Autodesk Inventor part; units mm, degrees
ref_plane "YZ Plane" through (0, 0, 0) normal (1, 0, 0) x (0, 1, 0)
ref_plane "XZ Plane" through (0, 0, 0) normal (0, 1, 0) x (-1, 0, 0)
ref_plane "XY Plane" through (0, 0, 0) normal (0, 0, 1) x (1, 0, 0)
sketch "Sketch1" plane through (0, 0, 0) normal (0, 0, 1) x (1, 0, 0)
  line L0 (8, 0.0718) -> (2, 3.5359)
  line L1 (2, 3.5359) -> (2, 10.4641)
  line L2 (2, 10.4641) -> (8, 13.9282)
  line L3 (8, 13.9282) -> (14, 10.4641)
  line L4 (14, 10.4641) -> (14, 3.5359)
  line L5 (14, 3.5359) -> (8, 0.0718)
  point P0 (0, 0)
  point P1 (8, 7)
  dimension "d1" = 12
extrude "Extrusion1" add sketch "Sketch1" along normal blind 18
sketch "Sketch2" plane through (0, 0, 0) normal (0, 0, -1) x (-1, 0, 0)
  circle A0 centre (-8, 7) radius 3.1
  point P0 (0, 0)
  dimension "d5" = 6.2
extrude "Extrusion2" cut sketch "Sketch2" against normal blind 14
sketch "Sketch3" plane through (0, 0, 18) normal (0, 0, 1) x (1, 0, 0)
  line L0 (14, 3.5359) -> (8, 0.0718)
  line L1 (14, 3.5359) -> (2, 3.5359)
  line L2 (2, 3.5359) -> (2, 10.4641)
  line L3 (2, 10.4641) -> (14, 10.4641)
  line L4 (14, 10.4641) -> (14, 3.5359)
  point P0 (0, 0)
  dimension "d12" = 6.9282
extrude "Extrusion3" add sketch "Sketch3" along normal blind 17
sketch "Sketch4" plane through (2, 10.4641, 18) normal (0, 1, 0) x (1, 0, 0)
  line L0 (12, 0) -> (12, -17)
  line L1 (12, -17) -> (15.5, -17)
  line L2 (0, 0) -> (0, -17)
  line L3 (12, 0) -> (12, -17)
  line L4 (0, -17) -> (-3.5, -17)
  line L5 (0, 0) -> (0, -17)
  line L6 (15.5, -17) -> (15.5, -3.1957)
  line L7 (-3.5, -3.1957) -> (0, 3.2792)
  line L8 (15.5, -3.1957) -> (12, 3.2792)
  line L9 (12, 18) -> (12, 0)
  line L10 (0, 0) -> (0, 3.2792)
  line L11 (12, 0) -> (12, 3)
  line L12 (-3.5, -17) -> (-3.5, -3.1957)
  point P0 (-2, 18)
  dimension "d10" = 3.5
  dimension "d11" = 3.5
extrude "Extrusion4" add sketch "Sketch4" against normal blind 6.9282
sketch "Sketch5" plane through (2, 10.4641, 18) normal (0, 1, 0) x (1, 0, 0)
  line L0 (15.5, -17) -> (15.5, -17)
  line L1 (0, -17) -> (12, -17)
  line L2 (12, -17) -> (12, -1)
  line L3 (12, -1) -> (0, -1)
  line L4 (0, -1) -> (0, -17)
  point P0 (-2, 18)
  point P1 (-3.5, -17)
extrude "Extrusion5" cut sketch "Sketch5" against normal through all
sketch "Sketch6" plane through (-1.5, 10.4641, 21.1957) normal (-1, 0, 0) x (0, 0, 1)
  line L0 (13.8043, 0) -> (13.8043, -6.9282)
  circle A0 centre (7.8043, -3.4641) radius 1.5
  point P0 (-21.1957, -10.4641)
  dimension "d18" = 3
extrude "Extrusion6" cut sketch "Sketch6" against normal through all
sketch "Sketch7" plane through (2, 3.5359, 18) normal (0, -1, 0) x (1, 0, 0)
  line L0 (-3.5, 12.5) -> (0, 12.5)
  line L1 (-3.5, 12.5) -> (-1.7726, 17)
  line L2 (0, 17) -> (-3.5, 17)
  line L3 (-3.5, 12.5) -> (1.3202, 12.5) construction
  line L4 (-3.5, 3.1957) -> (-3.5, 17)
  line L5 (-3.5, 12.5) -> (-3.5, 17)
  line L6 (-3.5, 17) -> (-1.7726, 17)
  line L7 (15.5, 12.9998) -> (19.7846, 12.9998) construction
  line L8 (15.5, 12.9998) -> (13.75, 17)
  line L9 (15.5, 17) -> (12, 17)
  line L10 (13.7726, 17) -> (15.5, 17)
  line L11 (15.5, 17) -> (15.5, 12.9998)
  line L12 (-3.5, 17) -> (-3.5, 12.5)
  line L13 (-3.5, 12.5) -> (-1.7726, 17)
  line L14 (-3.5, 17) -> (-3.5, 12.5)
  point P0 (-2, -18)
  dimension "d21" = 69
  dimension "d23" = 1.7274
  dimension "d24" = 1.7274
extrude "Extrusion7" cut sketch "Sketch7" against normal through all
properties part number "supportrodv2"
Check sheet for the modelled part. Datum: model origin and axes. Units: mm. A direction names the side the tool comes from. Coordinates: 2 decimals unless noted, no trailing zeros. Loops run counter-clockwise (first coordinate to the right, second up) from the corner with the lowest first, then second, coordinate; pieces in that order, holes last. Notation, with made-up numbers: (-5.75, 24.5) -> (2.25, 24.5) arc R20 cw to (2.25, 63.5) -> close; hole circle Ø11 at (56.5, 58). An arc over 180 degrees is marked (long way). Write item = value, one per line. Start each with the question number.
1. Section check D-D on z = 11.5. Record the cut outline in (x, y), then the cut area to 3 significant figures.
2. Section check A-A on z = 29. Record the cut outline in (x, y).
3. Material ranges on line 1 (Y direction, x = -0.65, z = 29); line 2 (Z direction, x = 11.25, y = 9); line 3 (Z direction, x = 6.75, y = 11.25), recorded low to high.
4. Section check C-C on z = 24.5. Record the cut outline in (x, y).
5. Depth check by flat-ended pin: P1, Ø6, axis at x = 0.5, z = 31, coming from the -Y side; P2, Ø1.8, axis at y = 7, z = 29, coming from the -X side; P3, Ø5, axis at y = 5.5, z = 8, coming from the -X side; P4, Ø1.7, axis at x = 6.5, y = 1.5, coming from the +Z side. Enter the tip coordinate at first touch or a pass-through.
6. Draft check along Y on faces 1 (the cylindrical face through (15.73, 7.07, 27.5)), 2 (the flat face through (5.04, 1.78, 8.87)), 3 (the flat face through (15.774, 7.048, 18.004)), 4 (the flat face through (8, 7, 14)). Enter one of: released by +Y, released by -Y, zero draft, split by the parting line, or undercut.
7. Section check B-B on y = 6.5. Record the cut outline in (x, z).
8. Tool access check on faces 5 (the flat face through (2, 7, 7)), 6 (the flat face through (8, 12, 18)), 7 (the flat face through (8, 2, 18)), 8 (the flat face through (14, 7, 7)), 9 (the flat face through (2, 7, 27)). Record the directions out of +Z, -Z, +X, -X, +Y, -Y that give a thin tool (end or side, any length) a straight path to the whole face; none if there is none.
Responses:
q1.outline = (2, 3.54) -> (8, 0.07) -> (14, 3.54) -> (14, 10.46) -> (8, 13.93) -> (2, 10.46) -> close; hole circle Ø6.2 at (8, 7)
q1.area = 94.5 mm2
q2.outline = (-1.5, 3.54) -> (2, 3.54) -> (2, 5.5) -> (-1.5, 5.5) -> close; (-1.5, 8.5) -> (2, 8.5) -> (2, 10.46) -> (-1.5, 10.46) -> close; (14, 3.54) -> (17.5, 3.54) -> (17.5, 5.5) -> (14, 5.5) -> close; (14, 8.5) -> (17.5, 8.5) -> (17.5, 10.46) -> (14, 10.46) -> close
q3.line_1 = 3.54 to 5.5, 8.5 to 10.46
q3.line_2 = 0 to 19
q3.line_3 = 0 to 18
q4.outline = (-1.5, 3.54) -> (2, 3.54) -> (2, 10.46) -> (-1.5, 10.46) -> close; (14, 3.54) -> (17.5, 3.54) -> (17.5, 10.46) -> (14, 10.46) -> close
q5.P1 = 3.54
q5.P2 = through
q5.P3 = 2
q5.P4 = 18
q6.face_1 = undercut
q6.face_2 = released by -Y
q6.face_3 = zero draft
q6.face_4 = undercut
q7.outline = (-1.5, 21.2) -> (2, 14.72) -> (2, 0) -> (4.94, 0) -> (4.94, 14) -> (11.06, 14) -> (11.06, 0) -> (14, 0) -> (14, 14.72) -> (17.5, 21.2) -> (17.5, 27.59) -> (14, 27.59) -> (14, 19) -> (2, 19) -> (2, 27.59) -> (-1.5, 27.59) -> close; (-1.5, 30.41) -> (2, 30.41) -> (2, 35) -> (0.23, 35) -> (-1.5, 30.5) -> close; (14, 30.41) -> (17.5, 30.41) -> (17.5, 31) -> (15.75, 35) -> (14, 35) -> close
q8.face_5 = -Z, -X, +Y, -Y
q8.face_6 = +Z, +X, -X, +Y
q8.face_7 = +Z, +X, -X, -Y
q8.face_8 = -Z, +X, +Y, -Y
q8.face_9 = +Z, +Y, -Y
